```python
from build123d import *

# Parameters (mm, degrees)
F1_DEPTH = 55
F3_DEPTH = 20


with BuildPart() as f1:
    # F0 (on Front) → F1 (new body)
    with BuildSketch(Plane.XZ):
        Polygon((-22.45298, 20), (-22.45298, 0), (52.54702, 0), align=None)
    extrude(amount=F1_DEPTH)

    # F2 (on Top) → F3 (cut)
    with BuildSketch(Plane.XY):
        Polygon((-22.493402, 0), (-22.493402, -55), (5.006598, -27.5), align=None)
    extrude(amount=F3_DEPTH, mode=Mode.SUBTRACT)


solid = f1.part
```
Input: part model. Units: mm. Frame: model coordinates. A direction names the side the tool comes from. Round coordinates to 2 decimals unless told otherwise and drop trailing zeros. Loops run counter-clockwise (first coordinate to the right, second up) from the corner with the lowest first, then second, coordinate; pieces in that order, holes last. Notation, with made-up numbers: (78, 47.25) -> (88, 47.25) arc R8 cw to (88, 53.25) -> close; hole circle Ø9 at (-35.75, -21). An arc over 180 degrees is marked (long way). One line per item, written item: value.
(1) Section D-D (y = -3). Return the cut outline in (x, z).
Geometry check:
outline: (-19.49, 0) -> (52.55, 0) -> (-19.49, 19.21) -> close
(2) Section C-C (z = 2.5). Return the cut outline in (x, y), plus the area to 3 significant figures.
Geometry check:
outline: (-22.45, -55) -> (43.17, -55) -> (43.17, 0) -> (-22.45, 0) -> (-22.45, -0.04) -> (5.01, -27.5) -> (-22.45, -54.96) -> close
area: 2,860 mm2
(3) Material intervals for line 1 (Y direction, x = -6, z = 7.5); line 2 (Y direction, x = -17, z = 18.5); line 3 (Z direction, x = 39, y = -27), sorted ascending. Write a range as [from, to].
Geometry check:
line 1: [-55, -38.51], [-16.49, 0]
line 2: [-55, -49.51], [-5.49, 0]
line 3: [0, 3.61]
(4) Pin query (flat end, axial travel): pin 1 (12 mm diameter, centred on y = -40.5, z = 10.5, fed in from -X). Return the tip coordinate at first contact, or that it passes through.
Geometry check:
pin 1: x = -13.99
(5) Section B-B (z = 18.5). Return the cut outline in (x, y).
Geometry check:
outline: (-22.45, -55) -> (-16.83, -55) -> (-16.83, -49.33) -> (-22.45, -54.96) -> close; (-22.45, -0.04) -> (-16.83, -5.67) -> (-16.83, 0) -> (-22.45, 0) -> close
(6) Mould query, pull axis Y, two halves, no side actions, for faces 3 (the face through (-2, 0, 6)), 4 (the face through (-8.531, -13.962, 7.638)), 5 (the face through (23.905, -27.115, 7.638)). Classes: pulls with the +Y half, pulls with the -Y half, needs draft (parallel to the pull), parting line crosses it, or undercut.
Geometry check:
face 3: pulls with the +Y half
face 4: undercut
face 5: needs draft
(7) Set-up query: faces 1 (the face through (-8.915, -41.422, 7.638)), 2 (the face through (23, -27, 0)). Return all of +Z, -Z, +X, -X, +Y, -Y with unobstructed straight access to the full face (end or side cutting, diameter ignored); none if empty.
Geometry check:
face 1: +Z, -Z, -X
face 2: -Z, +X, -X, +Y, -Y
(8) Section A-A (x = -7). Return the cut outline in (y, z), plus the area to 3 significant figures.
Geometry check:
outline: (-55, 0) -> (-39.51, 0) -> (-39.51, 15.88) -> (-55, 15.88) -> close; (-15.49, 0) -> (0, 0) -> (0, 15.88) -> (-15.49, 15.88) -> close
area: 492 mm2
